Design review of the part built by this model. Coordinates are the model's own, in mm. A direction names the side the tool comes from. Coordinates: 2 decimals unless noted, no trailing zeros. Order: outer loops, then holes, each group sorted by start corner. A loop starts at its lowest first (then second) coordinate and runs counter-clockwise, first axis right, second up. Notation, with made-up numbers: (54.25, 55) -> (84.25, 55) arc R24 cw to (84.25, 84) -> close; hole circle Ø11 at (31, -14). An arc over 180 degrees is marked (long way). Write item = value, one per line.
Autodesk Inventor part; units mm, degrees
ref_plane "YZ Plane" through (0, 0, 0) normal (1, 0, 0) x (0, 1, 0)
ref_plane "XZ Plane" through (0, 0, 0) normal (0, 1, 0) x (-1, 0, 0)
ref_plane "XY Plane" through (0, 0, 0) normal (0, 0, 1) x (1, 0, 0)
sketch "Sketch1" plane through (0, 0, 0) normal (0, 0, 1) x (1, 0, 0)
  circle A0 centre (0, 0) radius 19.175
  dimension "d0" = 38.35
extrude "Extrusion1" add sketch "Sketch1" along normal blind 24.81
sketch "Sketch2" plane through (0, 0, 24.81) normal (0, 0, 1) x (1, 0, 0)
  circle A0 centre (0, 0) radius 19.175
  line L0 (-31.75, 19.175) -> (31.75, 19.175)
  line L1 (31.75, 19.175) -> (31.75, -19.175)
  line L2 (31.75, -19.175) -> (-31.75, -19.175)
  line L3 (-31.75, -19.175) -> (-31.75, 19.175)
  point P0 (0, -19.175)
  dimension "d3" = 63.5
extrude "Extrusion2" add sketch "Sketch2" along normal blind 18.9
sketch "Sketch3" plane through (0, 0, 0) normal (0, 0, -1) x (-1, 0, 0)
  circle A0 centre (0, 0) radius 19.175
  line L0 (-15, 0) -> (15, 0)
  dimension "d6" = 30
hole "Hole1" at (15, 0, 0) at (-15, 0, 0) direction (0, 0, 1) diameter 3.302 depth 12.7 tip angle 118
sketch "Sketch4" plane through (-31.75, -19.175, 24.81) normal (-1, 0, 0) x (0, 0, 1)
  line L0 (18.9, 0) -> (18.9, 38.35)
  line L1 (18.9, 24.7099) -> (7.724, 24.7099)
  line L2 (7.724, 24.7099) -> (7.724, 12.0099)
  line L3 (7.724, 12.0099) -> (18.9, 12.0099)
  line L4 (18.9, 12.0099) -> (18.9, 24.7099)
  point P0 (-24.81, 19.175)
  dimension "d14" = 12.7
  dimension "d15" = 11.176
extrude "Extrusion3" cut sketch "Sketch4" against normal through all
properties part number "gripper" material "Aluminum-6061"
(1) We need section B-B (x = 25). Write out the cut boundary in (y, z) (3 decimals).
Report:
outline = (-19.175, 24.81) -> (19.175, 24.81) -> (19.175, 43.71) -> (5.535, 43.71) -> (5.535, 32.534) -> (-7.165, 32.534) -> (-7.165, 43.71) -> (-19.175, 43.71) -> close
(2) The part is to be moulded in two halves that separate along Y. For faces 1 (the flat face through (31.75, 0, 32)), 2 (the conical face through (15.28, -0.04, 13.52)), 3 (the cylindrical face through (-4.16, 18.72, 12.23)), 4 (the flat face through (0, 19.175, 34)), say which applies: released by +Y, released by -Y, zero draft, split by the parting line, or undercut.
Report:
face_1 = zero draft
face_2 = undercut
face_3 = split by the parting line
face_4 = released by +Y
(3) We need section D-D (z = 6.5). Write out the cut boundary in (x, y) (3 decimals).
Report:
outline = circle Ø38.35 at (0, 0); hole circle Ø3.302 at (-15, 0); hole circle Ø3.302 at (15, 0)
(4) We need section C-C (y = 9.5). Write out the cut boundary in (x, z).
Report:
outline = (-31.75, 24.81) -> (-16.66, 24.81) -> (-16.66, 0) -> (16.66, 0) -> (16.66, 24.81) -> (31.75, 24.81) -> (31.75, 43.71) -> (-31.75, 43.71) -> close
(5) For faces 5 (the flat face through (0, -19.175, 34)), 6 (the flat face through (0, 5.535, 38)), 7 (the cylindrical face through (16.6, -0.4, 6.4)), list the 3-axis set-ups (+Z, -Z, +X, -X, +Y, -Y) from which the entire face can be reached by the end or side of a thin tool; tool diameter is ignored.
Report:
face_5 = +Z, -Z, +X, -X, -Y
face_6 = +Z, +X, -X
face_7 = -Z
(6) Insertion check: pin 1 (9.5 mm diameter, centred on x = 23, y = 7, fed in from -Z); pin 2 (2.5 mm diameter, centred on x = -15, y = 0, fed in from -Z); pin 3 (6.5 mm diameter, centred on x = 15, y = -2, fed in from +Z); pin 4 (8 mm diameter, centred on y = -2.5, z = 33.5, fed in from -X). Each pin has a flat end and moves straight along its axis. Give the tip position at first contact, or say it passes through.
Report:
pin_1 = 24.81
pin_2 = 12.94
pin_3 = 32.53
pin_4 = -31.75
(7) For L1, parallel to X at y = 0, z = 7 (3 decimals); L2, parallel to X at y = 0.5, z = 7.5; L3, parallel to Y at x = -19, z = 39.5 (3 decimals), list the stretches that pass through material, from the lowest coordinate up.
Report:
L1 = -19.175 to -16.651, -13.349 to 13.349, 16.651 to 19.175
L2 = -19.17 to -16.57, -13.43 to 13.43, 16.57 to 19.17
L3 = -19.175 to -7.165, 5.535 to 19.175
(8) We need section A-A (z = 33.5). Write out the cut boundary in (x, y) (3 decimals), and give its area (3 significant figures).
Report:
outline = (-31.75, -19.175) -> (31.75, -19.175) -> (31.75, -7.165) -> (-31.75, -7.165) -> close; (-31.75, 5.535) -> (31.75, 5.535) -> (31.75, 19.175) -> (-31.75, 19.175) -> close
area = 1,630 mm²
